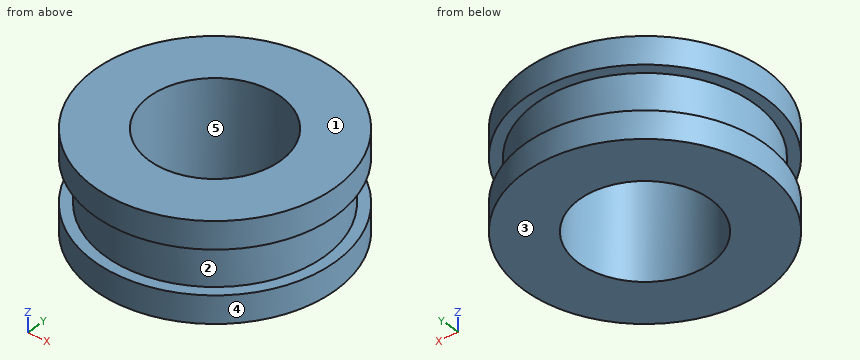
```python
from build123d import *

# Parameters (mm, degrees)
SKETCH_2_R          = 5.5
SKETCH_2_R_2        = 3
EXTRUDE_1_DEPTH     = 2.25
SKETCH_3_OUTSIDE_W  = 16.238
SKETCH_3_OUTSIDE_H  = 16.238
SKETCH_3_OUTSIDE_R  = 5
CUT_EXTRUDE_1_DEPTH = 1


with BuildPart() as part:
    # 草图2 → 凸台-拉伸1 (new, symmetric)
    with BuildSketch(Plane.XY):
        Circle(SKETCH_2_R)
        Circle(SKETCH_2_R_2, mode=Mode.SUBTRACT)
    extrude(amount=EXTRUDE_1_DEPTH, both=True)

    # 草图3 outside → 切除-拉伸1 (cut, symmetric)
    with BuildSketch(Plane.XY):
        Rectangle(SKETCH_3_OUTSIDE_W, SKETCH_3_OUTSIDE_H)
        Circle(SKETCH_3_OUTSIDE_R, mode=Mode.SUBTRACT)
    extrude(amount=CUT_EXTRUDE_1_DEPTH, both=True, mode=Mode.SUBTRACT)


solid = part.part
```
Here's how the part is built. I have some questions about the finished solid (model axes, mm). Face numbers are marked on the shaded views. A direction names the side the tool comes from. Round coordinates to 2 decimals unless told otherwise and drop trailing zeros. Loops run counter-clockwise (first coordinate to the right, second up) from the corner with the lowest first, then second, coordinate; pieces in that order, holes last.
1. Will these pins go through, and if not, where does the flat tip stop? pin 1 (1 mm diameter, centred on y = 3.5, z = 1.5, fed in from -X); pin 2 (2 mm diameter, centred on x = -3.5, z = -1, fed in from +Y).
Answers:
pin 1: stops at x = -4.61
pin 2: stops at y = 4.9
2. Thinking about a two-plate mould opening in Y: for the marked faces 3, 4 and 5, which applies, released by +Y, released by -Y, zero draft, split by the parting line, or undercut?
Answers:
face 3: zero draft
face 4: split by the parting line
face 5: undercut
3. For the marked faces 1 and 2, which set-ups out of +Z, -Z, +X, -X, +Y, -Y let a thin tool reach every point of the face, with its end or its side?
Answers:
face 1: +Z, +X, -X, +Y, -Y
face 2: none
4. If I drill on probe 1 along Y at (x, z) = (0, -0.4); probe 2 along Y at (x, z) = (0, 1.05); probe 3 along Z at (x, y) = (-4.75, -2), over which ranges is the centre line in solid material (lowest first)?
Answers:
probe 1: y = -5 to -3, 3 to 5
probe 2: y = -5.5 to -3, 3 to 5.5
probe 3: z = -2.25 to -1, 1 to 2.25
5. Suppose I cut it at D-D, the plane y = 3.75. Please give me the cut outline in (x, z), and give its area (3 significant figures).
Answers:
outline: (-4.02, -2.25) - (4.02, -2.25) - (4.02, -1) - (3.31, -1) - (3.31, 1) - (4.02, 1) - (4.02, 2.25) - (-4.02, 2.25) - (-4.02, 1) - (-3.31, 1) - (-3.31, -1) - (-4.02, -1) - close
area: 33.3 mm2
6. Suppose I cut it at C-C, the plane z = -1.9. Please give me the cut outline in (x, y), and give its area (3 significant figures).
Answers:
outline: circle Ø11 at (0, 0); hole circle Ø6 at (0, 0)
area: 66.8 mm2
7. Suppose I cut it at A-A, the plane y = 0. Please give me the cut outline in (x, z).
Answers:
outline: (-5.5, -2.25) - (-3, -2.25) - (-3, 2.25) - (-5.5, 2.25) - (-5.5, 1) - (-5, 1) - (-5, -1) - (-5.5, -1) - close; (3, -2.25) - (5.5, -2.25) - (5.5, -1) - (5, -1) - (5, 1) - (5.5, 1) - (5.5, 2.25) - (3, 2.25) - close
